```python
from build123d import *

# Parameters (mm, degrees)
EXTRUDE_1_DEPTH     = 40
SKETCH_2_W          = 25
SKETCH_2_H          = 47
EXTRUDE_2_DEPTH     = 40
HOLE_WIZARD_3_D     = 23
EXTRUDE_3_DEPTH     = 40
EXTRUDE_5_DEPTH     = 20
HOLE_WIZARD_4_D     = 5.2
SKETCH_15_R         = 3
CUT_EXTRUDE_1_DEPTH = 3
EXTRUDE_START       = 5
SKETCH_16_R         = 11.5
EXTRUDE_6_DEPTH     = 5


with BuildPart() as part:
    # 草图1 → 凸台-拉伸1 (new body)
    with BuildSketch(Plane.XY):
        Polygon((13.1, -5.375), (13.1, -25.375), (10.1, -25.375), (10.1, -5.375), (-10.1, -5.375), (-10.1, -25.375), (-13.1, -25.375), (-13.1, -5.375), (-25, -5.375), (-25, 5.375), (25, 5.375), (25, -5.375), align=None)
    extrude(amount=EXTRUDE_1_DEPTH)

    # 草图2 → 凸台-拉伸2 (add)
    with BuildSketch(Plane(origin=(0, 0, 0), x_dir=(-1, 0, 0), z_dir=(0, 0, -1))):
        with Locations((0, 28.875)):
            Rectangle(SKETCH_2_W, SKETCH_2_H)
    extrude(amount=-EXTRUDE_2_DEPTH)

    # 孔3 (through all)
    with Locations(Plane.XY.offset(40)):
        with Locations((0, 35.625)):
            Hole(HOLE_WIZARD_3_D / 2)

    # 草图10 → 凸台-拉伸3 (add)
    with BuildSketch(Plane.XY.offset(40)):
        Polygon((12.5, 35.375), (17.5, 35.375), (25, 15.375), (25, 5.375), (12.5, 5.375), align=None)
        Polygon((-12.5, 35.375), (-12.5, 5.375), (-25, 5.375), (-25, 15.375), (-17.5, 35.375), align=None)
    extrude(amount=-EXTRUDE_3_DEPTH)

    # 草图12 → 凸台-拉伸5 (add)
    with BuildSketch(Plane.XY.offset(40)):
        Polygon((12.5, 52.375), (17.5, 35.375), (12.5, 35.375), align=None)
        Polygon((-12.5, 52.375), (-17.5, 35.375), (-12.5, 35.375), align=None)
    extrude(amount=-EXTRUDE_5_DEPTH)

    # 孔4 (through all)
    with Locations(Plane(origin=(13.1, 0, 0), x_dir=(0, 0, -1), z_dir=(1, 0, 0))):
        with Locations((-31, -15.375), (-9, -15.375)):
            Hole(HOLE_WIZARD_4_D / 2)

    # 草图15 → 切除-拉伸1 (cut)
    with BuildSketch(Plane.XY.offset(40)):
        with Locations((-15.5, 51.125)):
            Circle(SKETCH_15_R)
        with Locations((15.5, 51.125)):
            Circle(SKETCH_15_R)
        with Locations((-15.5, 20.125)):
            Circle(SKETCH_15_R)
        with Locations((15.5, 20.125)):
            Circle(SKETCH_15_R)
    extrude(amount=-CUT_EXTRUDE_1_DEPTH, mode=Mode.SUBTRACT)

    # 草图16 → 凸台-拉伸6 (add)
    with BuildSketch(Plane(origin=(0, 0, 0), x_dir=(-1, 0, 0), z_dir=(0, 0, -1)).offset(EXTRUDE_START)):
        Polygon((-25, 3.625), (25, 3.625), (25, 15.375), (17.5, 35.375), (12.5, 35.375), (12.5, 52.375), (-12.5, 52.375), (-12.5, 35.375), (-17.5, 35.375), (-25, 15.375), align=None)
        with Locations(Location((0, 35.625, 0), (0, 0, 180))):
            Circle(SKETCH_16_R, mode=Mode.SUBTRACT)
    extrude(amount=-EXTRUDE_6_DEPTH)


solid = part.part
```
Can you work these out from the model? Positions are in its coordinate system, mm. A direction names the side the tool comes from. Coordinates: 2 decimals unless noted, no trailing zeros. Order: outer loops, then holes, each group sorted by start corner. A loop starts at its lowest first (then second) coordinate and runs counter-clockwise, first axis right, second up. Notation, with made-up numbers: (-30, 67) -> (28, 67) arc R20 ccw to (28, 74) -> close; hole circle Ø7 at (10.25, 40.25). An arc over 180 degrees is marked (long way). Write each question's results on one line, items separated by ' | '.
Item 1: I want a section at A-A, the plane z = 29.5. Write out the boundary of the cut face in (x, y) (3 decimals), then the cut area to 3 significant figures.
Results are:
outline: (-25, -5.375) -> (-13.1, -5.375) -> (-13.1, -13.251) -> (-10.1, -13.251) -> (-10.1, -5.375) -> (10.1, -5.375) -> (10.1, -13.251) -> (13.1, -13.251) -> (13.1, -5.375) -> (25, -5.375) -> (25, 15.375) -> (17.5, 35.375) -> (12.5, 52.375) -> (-12.5, 52.375) -> (-17.5, 35.375) -> (-25, 15.375) -> close; (-13.1, -25.375) -> (-10.1, -25.375) -> (-10.1, -17.499) -> (-13.1, -17.499) -> close; (10.1, -25.375) -> (13.1, -25.375) -> (13.1, -17.499) -> (10.1, -17.499) -> close; hole circle Ø23 at (0, 35.625) | area: 2,080 mm²
Item 2: If we mould it in two halves opening along Z, with no side actions, what happens to faces 1 (the face through (14, 40, 20)), 2 (the face through (11.58, -16.96, 28.94)), 3 (the face through (-17.88, 18.3, 38.52))? For each: +Z half, -Z half, draft (parallel to the pull), parting line (faces both ways), or undercut.
Results are:
face 1: -Z half | face 2: undercut | face 3: draft
Item 3: I want a section at B-B, the plane y = 32.5. Write out the boundary of the cut face in (x, z), then the cut area to 3 significant figures.
Results are:
outline: (-18.58, -5) -> (-11.07, -5) -> (-11.07, 40) -> (-18.58, 40) -> close; (11.07, -5) -> (18.58, -5) -> (18.58, 40) -> (11.07, 40) -> close | area: 676 mm²
Item 4: I want a section at C-C, the plane x = -3.5. Write out the boundary of the cut face in (y, z) (3 decimals).
Results are:
outline: (-5.375, 0) -> (3.625, 0) -> (3.625, -5) -> (24.671, -5) -> (24.671, 40) -> (-5.375, 40) -> close; (46.579, -5) -> (52.375, -5) -> (52.375, 40) -> (46.579, 40) -> close
Item 5: Which directions (+Z, -Z, +X, -X, +Y, -Y) give clear straight access to the entire face, cutting with the end or side of a thin tool? Please do faces 4 (the face through (13.1, -15, 20)), 5 (the face through (12.615, 50.302, 38.521)), 6 (the face through (-12.629, 50.256, 38.521)), 7 (the face through (-19, -5.375, 20)).
Results are:
face 4: +Z, -Z, +X, -Y | face 5: +Z, +X | face 6: +Z, -X | face 7: +Z, -Z, -X, -Y
Item 6: If I drill on line 1 along X through (y, z) = (-10, 21); line 2 along Y through (x, z) = (-11.65, 9) (3 decimals); line 3 along Y through (x, z) = (0, -2) (3 decimals), over which ranges is the centre line in solid material (lowest first)?
Results are:
line 1: -13.1 to -10.1, 10.1 to 13.1 | line 2: -25.375 to -17.975, -12.775 to 52.375 | line 3: 3.625 to 24.125, 47.125 to 52.375
Item 7: I want a section at D-D, the plane z = 22.5. Write out the boundary of the cut face in (x, y) (3 decimals), then the cut area to 3 significant figures.
Results are:
outline: (-25, -5.375) -> (-13.1, -5.375) -> (-13.1, -25.375) -> (-10.1, -25.375) -> (-10.1, -5.375) -> (10.1, -5.375) -> (10.1, -25.375) -> (13.1, -25.375) -> (13.1, -5.375) -> (25, -5.375) -> (25, 15.375) -> (17.5, 35.375) -> (12.5, 52.375) -> (-12.5, 52.375) -> (-17.5, 35.375) -> (-25, 15.375) -> close; hole circle Ø23 at (0, 35.625) | area: 2,100 mm²
Item 8: I'm going to push flat-ended pins straight in: pin 1 Ø1.8 at (x, y) = (14.5, 20) entering from +Z; pin 2 Ø6 at (y, z) = (-13, 17.5) entering from +X; pin 3 Ø4.5 at (y, z) = (-15.375, 31) entering from +X; pin 4 Ø6 at (y, z) = (20, 12) entering from +X. Where does each tip first touch, or does it pass through?
Results are:
pin 1: z = 37 | pin 2: x = 13.1 | pin 3: through | pin 4: x = 24.39
